Design review of the part built by this model. Coordinates are the model's own, in mm. Face numbers are marked on the shaded views. A direction names the side the tool comes from. Give positions to 0.01 mm unless a question says otherwise; leave off trailing zeros. Loops run counter-clockwise (first coordinate to the right, second up) from the corner with the lowest first, then second, coordinate; pieces in that order, holes last. Notation, with made-up numbers: (12.5, 36) - (16.5, 36) arc R21 ccw to (16.5, 58) - close; hole circle Ø5 at (4.5, -4.75). An arc over 180 degrees is marked (long way). One line per item, written item: value. Start each with the question number.
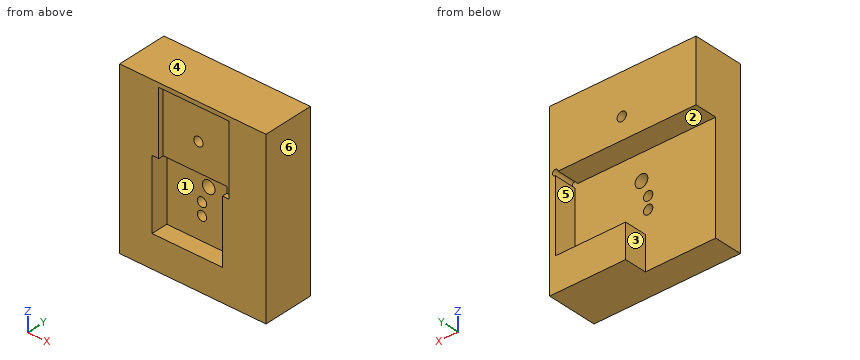
```python
from build123d import *

# Parameters (mm, degrees)
SKETCH_1_W                = 50
SKETCH_1_H                = 26.71
EXTRUDE_1_DEPTH           = 6
EXTRUDE_2_DEPTH           = 8
EXTRUDE_2_DEPTH_BACK      = 6
HOLE_WIZARD_M4_1_D        = 3.3
HOLE_WIZARD_M4_1_DEPTH    = 10.1
HOLE_WIZARD_M4_1_TIP      = 0.991420021
SKETCH_12_W               = 2
SKETCH_12_H               = 8
CUT_EXTRUDE_5_DEPTH       = 25
EXTRUDE_5_DEPTH           = 10
SKETCH_25_W               = 52
SKETCH_25_H               = 14
EXTRUDE_6_DEPTH           = 20
SKETCH_13_R               = 1
CUT_EXTRUDE_6_DEPTH       = 8
SKETCH_5_W                = 25
SKETCH_5_H                = 25
SKETCH_5_R                = 1.193891983
CUT_EXTRUDE_1_DEPTH       = 2
HOLE_WIZARD_M4_2_D        = 3.3
SKETCH_14_W               = 52
SKETCH_14_H               = 60.71
SKETCH_14_W_2             = 25
SKETCH_14_H_2             = 25
EXTRUDE_3_DEPTH           = 4
SKETCH_16_W               = 25
SKETCH_16_H               = 25
CUT_EXTRUDE_7_DEPTH       = 1.84
HOLE_WIZARD_0_D           = 4.5
HOLE_WIZARD_0_CBORE_D     = 8
HOLE_WIZARD_0_CBORE_DEPTH = 4.6
HOLE_WIZARD_M4_3_D        = 3.3


with BuildPart() as part:
    # 草图1 → 凸台-拉伸1 (new body)
    with BuildSketch(Plane(origin=(0, 0, 0), x_dir=(1, 0, 0), z_dir=(0, 1, 0))):
        Rectangle(SKETCH_1_W, SKETCH_1_H)
    extrude(amount=EXTRUDE_1_DEPTH)

    # 草图2 → 凸台-拉伸2 (add, two sides: drawn at the far end of the back side and taken through both)
    with BuildSketch(Plane(origin=(0, 6, 0), x_dir=(1, 0, 0), z_dir=(0, 1, 0)).offset(-EXTRUDE_2_DEPTH_BACK)):
        Polygon((25, 13.355), (-25, 13.355), (-25, 15.355), (27, 15.355), (27, -15.355), (-25, -15.355), (-25, -13.355), (25, -13.355), align=None)
    extrude(amount=EXTRUDE_2_DEPTH + EXTRUDE_2_DEPTH_BACK)

    # M4 螺纹孔1
    with Locations(Plane(origin=(-1, 6, -5.855), x_dir=(0, 0, 1), z_dir=(0, 1, 0))):
        with Locations((0, 0)):
            Hole(HOLE_WIZARD_M4_1_D / 2, depth=HOLE_WIZARD_M4_1_DEPTH)
            with Locations((0, 0, -(HOLE_WIZARD_M4_1_DEPTH + HOLE_WIZARD_M4_1_TIP / 2))):  # 118° drill point
                Cone(0, HOLE_WIZARD_M4_1_D / 2, HOLE_WIZARD_M4_1_TIP, mode=Mode.SUBTRACT)

    # 草图12 → 切除-拉伸5 (cut)
    with BuildSketch(Plane.ZY.offset(25)):
        with Locations((-14.355, 10)):
            Rectangle(SKETCH_12_W, SKETCH_12_H)
    extrude(amount=-CUT_EXTRUDE_5_DEPTH, mode=Mode.SUBTRACT)

    # 草图24 → 凸台-拉伸5 (add)
    with BuildSketch(Plane(origin=(0, 0, -15.355), x_dir=(-1, 0, 0), z_dir=(0, 0, -1))):
        Polygon((25, 6), (0, 6), (0, 14), (-27, 14), (-27, 0), (25, 0), align=None)
    extrude(amount=EXTRUDE_5_DEPTH)

    # 草图25 → 凸台-拉伸6 (add)
    with BuildSketch(Plane.XY.offset(15.355)):
        with Locations((1, 7)):
            Rectangle(SKETCH_25_W, SKETCH_25_H)
    extrude(amount=EXTRUDE_6_DEPTH)

    # 草图13 → 切除-拉伸6 (cut)
    with BuildSketch(Plane(origin=(0, 14, 0), x_dir=(1, 0, 0), z_dir=(0, 1, 0))):
        with Locations((25, -13.355)):
            Circle(SKETCH_13_R)
    extrude(amount=-CUT_EXTRUDE_6_DEPTH, mode=Mode.SUBTRACT)

    # 草图5 → 切除-拉伸1 (cut)
    with BuildSketch(Plane.XZ):
        with Locations((-1, -1.455)):
            Rectangle(SKETCH_5_W, SKETCH_5_H)
        with Locations(Location((-1, -1.455, 0), (0, 0, 270))):
            Circle(SKETCH_5_R, mode=Mode.SUBTRACT)
    extrude(amount=-CUT_EXTRUDE_1_DEPTH, mode=Mode.SUBTRACT)

    # M4 螺纹孔2 (through all)
    with Locations(Plane(origin=(-1, 2, -1.455), x_dir=(0, 0, -1), z_dir=(0, -1, 0))):
        with Locations((0, 0)):
            Hole(HOLE_WIZARD_M4_2_D / 2)

    # 草图14 → 凸台-拉伸3 (add)
    with BuildSketch(Plane.XZ):
        with Locations((1, 5)):
            Rectangle(SKETCH_14_W, SKETCH_14_H)
        with Locations((-1, -1.455)):
            Rectangle(SKETCH_14_W_2, SKETCH_14_H_2, mode=Mode.SUBTRACT)
    extrude(amount=EXTRUDE_3_DEPTH)

    # 草图16 → 切除-拉伸7 (cut)
    with BuildSketch(Plane.XZ.offset(4)):
        with Locations((1.38, 21.365)):
            Rectangle(SKETCH_16_W, SKETCH_16_H)
    extrude(amount=-CUT_EXTRUDE_7_DEPTH, mode=Mode.SUBTRACT)

    # 打孔尺寸(%根据)内六角圆柱头螺钉的类型0 (through all)
    with Locations(Plane(origin=(1.378, -4, 4.369489244), x_dir=(0, 0, -1), z_dir=(0, -1, 0))):
        with Locations((0, 0)):
            CounterBoreHole(HOLE_WIZARD_0_D / 2, HOLE_WIZARD_0_CBORE_D / 2, HOLE_WIZARD_0_CBORE_DEPTH)

    # M4 螺纹孔3 (through all)
    with Locations(Plane(origin=(1.38, -2.16, 21.015906409), x_dir=(0, 0, -1), z_dir=(0, -1, 0))):
        with Locations((0, 0)):
            Hole(HOLE_WIZARD_M4_3_D / 2)


solid = part.part
```
(1) For pin 1 Ø2 at (x, z) = (10.5, -8.5) entering from +Y; pin 2 Ø12.5 at (x, z) = (0.5, 22) entering from -Y; pin 3 Ø2.5 at (x, z) = (25, 13.355) entering from +Y; pin 4 Ø6.5 at (y, z) = (12, -5.5) entering from -X, all flat-tipped, find the tip position at first contact; note any pin that passes through.
(2) Take a section at C-C on z = -11.5. State the section outline as (x, y) points.
(3) Machinability: for the marked faces 1, 2 and 3, which of the approach directions +Z, -Z, +X, -X, +Y, -Y give a long, thin tool a straight path to every point of the face, cutting with its end or side? Answer none if there is none.
(4) Draft analysis for pull direction Z (two halves, no side actions). For the marked faces 4, 5 and 6, state which applies: pulls with the +Z half, pulls with the -Z half, needs draft (parallel to the pull), parting line crosses it, or undercut.
(5) Take a section at A-A on y = 7.25. State the section outline as (x, z) points (3 decimals).
(6) Take a section at D-D on x = -6.5. State the section outline as (y, z) points (3 decimals), and give its area (3 significant figures).
(7) Take a section at B-B on x = 6. State the section outline as (y, z) points (3 decimals), and give its area (3 significant figures).
(8) To check wall thickness, follow L1, parallel to X at y = -0.75, z = 3.5; L2, parallel to X at y = 7.75, z = 13.5; L3, parallel to Y at x = 16, z = 2. State the ranges of each line that lie inside material, in increasing order. Write a range as from..to.
Here are the results:
1. pin 1: y = 6
1. pin 2: y = -2.16
1. pin 3: y = 14
1. pin 4: x = 25
2. outline: (-25, -4) - (-13.5, -4) - (-13.5, 2) - (11.5, 2) - (11.5, -4) - (27, -4) - (27, 14) - (25, 14) - (25, 6) - (-25, 6) - close
3. face 1: -Y
3. face 2: -X, +Y
3. face 3: -Z, -X, +Y
4. face 4: pulls with the +Z half
4. face 5: undercut
4. face 6: needs draft
5. outline: (-25, 13.355) - (24, 13.355) arc R1 cw (long way) to (25, 12.355) - (25, -13.355) - (0, -13.355) - (0, -25.355) - (27, -25.355) - (27, 35.355) - (-25, 35.355) - close; hole circle Ø3.3 at (1.38, 21.016)
6. outline: (-4, -25.355) - (6, -25.355) - (6, 13.355) - (14, 13.355) - (14, 35.355) - (-4, 35.355) - (-4, 33.865) - (-2.16, 33.865) - (-2.16, 11.045) - (2, 11.045) - (2, -13.955) - (-4, -13.955) - close
6. area: 591 mm²
7. outline: (-4, -25.355) - (14, -25.355) - (14, -13.355) - (6, -13.355) - (6, 13.355) - (14, 13.355) - (14, 35.355) - (-4, 35.355) - (-4, 33.865) - (-2.16, 33.865) - (-2.16, 11.045) - (2, 11.045) - (2, -13.955) - (-4, -13.955) - close
7. area: 687 mm²
8. L1: -25..-13.5, 11.5..27
8. L2: -25..24.01, 25.99..27
8. L3: -4..6
